Build history of the part. All positions in model axes, mm. Coordinates: 2 decimals unless noted, no trailing zeros. Order: outer loops, then holes, each group sorted by start corner. A loop starts at its lowest first (then second) coordinate and runs counter-clockwise, first axis right, second up. Notation, with made-up numbers: (38, 1) - (74, 1) arc R25 ccw to (74, 36) - close; hole circle Ø7 at (62, 57). An arc over 180 degrees is marked (long way). Write each question's results on one line, items separated by ' | '. Start each with the question number.
from build123d import *

# Parameters (mm, degrees)
SKETCH2_W                   = 500
SKETCH2_H                   = 185
BASE_DEPTH                  = 4
SKETCH3_W                   = 20
SKETCH3_H                   = 4
TOP_HOLE_DEFINITION_DEPTH   = 267.593792126
TOP_HOLE_PATTERN_COUNT      = 5
TOP_HOLE_PATTERN_PITCH      = 55
TOP_HOLE_PATTERN_COL_COUNT  = 5
TOP_HOLE_PATTERN_COL_PITCH  = 55
SKETCH4_W                   = 4
SKETCH4_H                   = 20
LEFT_HOLE_DEFINITION_DEPTH  = 267.593792126
LEFT_HOLE_PATTERN_COUNT     = 2
LEFT_HOLE_PATTERN_PITCH     = 55
LEFT_HOLE_PATTERN_COL_COUNT = 2
LEFT_HOLE_PATTERN_COL_PITCH = 55
FILLET1_R                   = 10
MIRROR2_COPY_1_SKETCH_W     = 4
MIRROR2_COPY_1_SKETCH_H     = 20
MIRROR2_COPY_1_DEPTH        = 267.593792126
MIRROR2_COPY_2_SKETCH_W     = 4
MIRROR2_COPY_2_SKETCH_H     = 20
MIRROR2_COPY_2_DEPTH        = 267.593792126
SKETCH7_R                   = 8
SKETCH7_R_2                 = 10
CUT_EXTRUDE5_DEPTH          = 267.593792126
SKETCH8_W                   = 27
SKETCH8_H                   = 16.8
CUT_EXTRUDE6_DEPTH          = 267.593792126


with BuildPart() as part:
    # Sketch2 → Base (new body)
    with BuildSketch(Plane(origin=(0, 0, 0), x_dir=(1, 0, 0), z_dir=(0, 1, 0))):
        Rectangle(SKETCH2_W, SKETCH2_H)
    extrude(amount=BASE_DEPTH)

    # Sketch3 → Top Hole Definition (cut, through all)
    with BuildSketch(Plane(origin=(0, 4, 0), x_dir=(1, 0, 0), z_dir=(0, 1, 0))):
        with Locations((0, 85.5)):
            Rectangle(SKETCH3_W, SKETCH3_H)
    top_hole_definition = extrude(amount=-TOP_HOLE_DEFINITION_DEPTH, mode=Mode.SUBTRACT)

    # Top Hole Pattern: Top Hole Definition ×5
    with Locations(*[(-i * TOP_HOLE_PATTERN_PITCH, 0, 0) for i in range(1, TOP_HOLE_PATTERN_COUNT)]):
        add(top_hole_definition, mode=Mode.SUBTRACT)

    # Top Hole Pattern col: Top Hole Definition ×5
    with Locations(*[(i * TOP_HOLE_PATTERN_COL_PITCH, 0, 0) for i in range(1, TOP_HOLE_PATTERN_COL_COUNT)]):
        add(top_hole_definition, mode=Mode.SUBTRACT)

    # Sketch4 → Left Hole Definition (cut, through all)
    with BuildSketch(Plane(origin=(0, 4, 0), x_dir=(1, 0, 0), z_dir=(0, 1, 0))):
        with Locations((-243, 0)):
            Rectangle(SKETCH4_W, SKETCH4_H)
    left_hole_definition = extrude(amount=-LEFT_HOLE_DEFINITION_DEPTH, mode=Mode.SUBTRACT)

    # Left Hole Pattern: Left Hole Definition ×2
    with Locations(*[(0, 0, -i * LEFT_HOLE_PATTERN_PITCH) for i in range(1, LEFT_HOLE_PATTERN_COUNT)]):
        add(left_hole_definition, mode=Mode.SUBTRACT)

    # Left Hole Pattern col: Left Hole Definition ×2
    with Locations(*[(0, 0, i * LEFT_HOLE_PATTERN_COL_PITCH) for i in range(1, LEFT_HOLE_PATTERN_COL_COUNT)]):
        add(left_hole_definition, mode=Mode.SUBTRACT)

    # Fillet1
    fillet1_edges = [part.edges().sort_by_distance(p)[0] for p in [
        (-250, 2, -92.5),
        (250, 2, -92.5),
        (250, 2, 92.5),
        (-250, 2, 92.5),
    ]]
    fillet(fillet1_edges, radius=FILLET1_R)

    # Mirror2: Left Hole Definition across plane
    add(left_hole_definition.mirror(Plane(origin=(0, 0, 0), x_dir=(0, 0, 1), z_dir=(1, 0, 0))), mode=Mode.SUBTRACT)

    # Mirror2 copy 1 sketch → Mirror2 copy 1 (cut, through all)
    with BuildSketch(Plane(origin=(0, 4, -55), x_dir=(-1, 0, 0), z_dir=(0, 1, 0))):
        with Locations((-243, 0)):
            Rectangle(MIRROR2_COPY_1_SKETCH_W, MIRROR2_COPY_1_SKETCH_H)
    extrude(amount=-MIRROR2_COPY_1_DEPTH, mode=Mode.SUBTRACT)

    # Mirror2 copy 2 sketch → Mirror2 copy 2 (cut, through all)
    with BuildSketch(Plane(origin=(0, 4, 55), x_dir=(-1, 0, 0), z_dir=(0, 1, 0))):
        with Locations((-243, 0)):
            Rectangle(MIRROR2_COPY_2_SKETCH_W, MIRROR2_COPY_2_SKETCH_H)
    extrude(amount=-MIRROR2_COPY_2_DEPTH, mode=Mode.SUBTRACT)

    # Sketch7 → Cut-Extrude5 (cut, through all)
    with BuildSketch(Plane.XZ):
        with Locations(Location((-209, 59.798294078, 0), (0, 0, 270))):
            Circle(SKETCH7_R)
        with Locations(Location((-168, 59.798294078, 0), (0, 0, 270))):
            Circle(SKETCH7_R)
        with Locations(Location((-127, 59.798294078, 0), (0, 0, 270))):
            Circle(SKETCH7_R)
        with Locations(Location((-86, 59.798294078, 0), (0, 0, 270))):
            Circle(SKETCH7_R)
        with Locations(Location((-45, 59.798294078, 0), (0, 0, 270))):
            Circle(SKETCH7_R)
        with Locations(Location((-4, 59.798294078, 0), (0, 0, 270))):
            Circle(SKETCH7_R)
        with Locations(Location((37, 59.798294078, 0), (0, 0, 270))):
            Circle(SKETCH7_R)
        with Locations(Location((78, 59.798294078, 0), (0, 0, 270))):
            Circle(SKETCH7_R)
        with Locations(Location((-179.5, 9.310158007, 0), (0, 0, 270))):
            Circle(SKETCH7_R_2)
        with Locations(Location((-209, 6.747125767, 0), (0, 0, 270))):
            Circle(SKETCH7_R)
        with Locations(Location((157.298294078, 61.5, 0), (0, 0, 270))):
            Circle(SKETCH7_R)
        with Locations(Location((157.431778922, 37.500371215, 0), (0, 0, 270))):
            Circle(SKETCH7_R)
        with Locations(Location((157.565263767, 13.500742431, 0), (0, 0, 270))):
            Circle(SKETCH7_R)
        with Locations(Location((157.698748611, -10.498886354, 0), (0, 0, 270))):
            Circle(SKETCH7_R)
    extrude(amount=-CUT_EXTRUDE5_DEPTH, mode=Mode.SUBTRACT)

    # Sketch8 → Cut-Extrude6 (cut, through all)
    with BuildSketch(Plane.XZ):
        with Locations((204.065263766, 59.1)):
            Rectangle(SKETCH8_W, SKETCH8_H)
    extrude(amount=-CUT_EXTRUDE6_DEPTH, mode=Mode.SUBTRACT)


solid = part.part
Item 1: Flat gauge pins, fed straight in: P1, Ø9.5, axis at x = 157.43, z = 37.5, coming from the -Y side; P2, Ø2, axis at x = 243.5, y = 2.5, coming from the +Z side; P3, Ø2, axis at y = 2.5, z = -85, coming from the +X side; P4, Ø1.2, axis at y = 1.5, z = -86, coming from the +X side. Where does each tip first touch, or does it go through?
Item 2: Pull direction X, two halves, no side cores. Call faces 1 (the cylindrical face through (-247.15, 2.03, -89.49)), 2 (the flat face through (-3, 0, -1)), 3 (the cylindrical face through (150.334, 1.972, 33.809)), 4 (the cylindrical face through (-1.597, 1.972, 52.168)): released by +X, released by -X, zero draft, split by the parting line, or undercut.
Item 3: Slice it at C-C (x = 202). Write the cut outline in (y, z).
Item 4: Slice it at A-A (x = -4). Write the cut outline in (y, z).
Item 5: Slice it at B-B (x = -127). Write the cut outline in (y, z).
Item 6: Slice it at D-D (y = 1). Count the separate pieces of the cut face and the enclosed holes in it, then the cut area to 3 significant figures.
Item 7: Probe probe 1 along Z at (x, y) = (113, 3); probe 2 along X at (y, z) = (0.9, 36); probe 3 along X at (y, z) = (0.65, 18.5). List the from-to ranges inside material, lowest first.
Resolved:
1) P1: through | P2: z = 92.18 | P3: x = 249.89 | P4: x = 249.57
2) face 1: released by -X | face 2: zero draft | face 3: undercut | face 4: undercut
3) outline: (0, -92.5) - (4, -92.5) - (4, 50.7) - (0, 50.7) - close; (0, 67.5) - (4, 67.5) - (4, 92.5) - (0, 92.5) - close
4) outline: (0, -92.5) - (4, -92.5) - (4, -87.5) - (0, -87.5) - close; (0, -83.5) - (4, -83.5) - (4, 51.8) - (0, 51.8) - close; (0, 67.8) - (4, 67.8) - (4, 92.5) - (0, 92.5) - close
5) outline: (0, -92.5) - (4, -92.5) - (4, 51.8) - (0, 51.8) - close; (0, 67.8) - (4, 67.8) - (4, 92.5) - (0, 92.5) - close
6) separate pieces: 1 | enclosed holes: 30 | area: 87,800 mm^2
7) probe 1: -92.5 to -87.5, -83.5 to 92.5 | probe 2: -250 to 149.57, 165.29 to 250 | probe 3: -250 to -183.44, -175.56 to 151.32, 163.81 to 250
